Geometry: see drawing. Coordinates: mm, zero at the bounding-box minimum. Coordinates: 2 decimals unless noted, no trailing zeros. Order: outer loops, then holes, each group sorted by start corner. A loop starts at its lowest first (then second) coordinate and runs counter-clockwise, first axis right, second up.
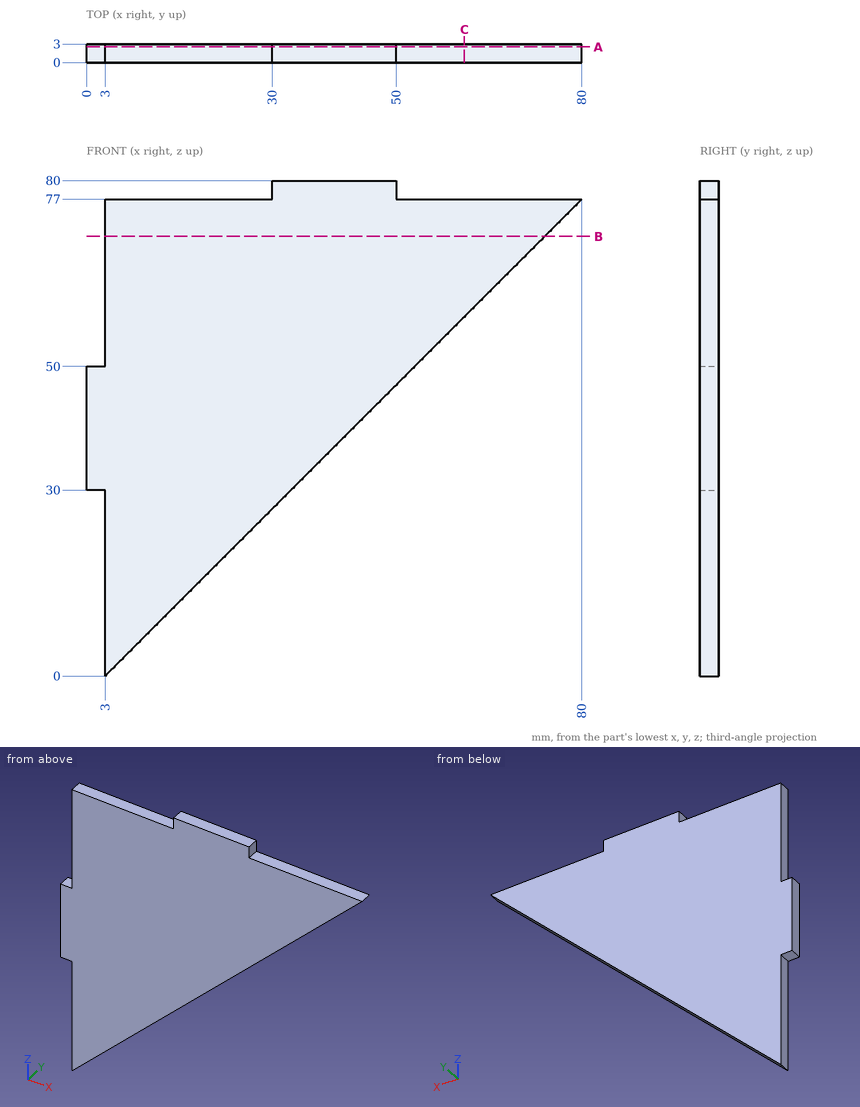
Q1. Section query C-C on x = 61. Output: boundary loops of the cut face in (y, z).
Solutions:
outline: (0, 58) - (3, 58) - (3, 77) - (0, 77) - close
Q2. Section query B-B on z = 71. Output: boundary loops of the cut face in (x, y).
Solutions:
outline: (3, 0) - (74, 0) - (74, 3) - (3, 3) - close
Q3. Pin query (flat end, axial travel): P1, Ø0.9, axis at y = 1, z = 78.5, coming from the +X side; P2, Ø1, axis at y = 0.5, z = 52.5, coming from the +X side; P3, Ø0.9, axis at x = 68.5, y = 1, coming from the +Z side. Return the tip coordinate at first contact, or that it passes through.
Solutions:
P1: stops at x = 50
P2: stops at x = 56
P3: stops at z = 77
Q4. Material intervals for line 1 along X through (y, z) = (2.5, 77.5); line 2 along Z through (x, y) = (36.5, 0.3); line 3 along X through (y, z) = (2.1, 38.5), sorted ascending.
Solutions:
line 1: x = 30 to 50
line 2: z = 33.5 to 80
line 3: x = 0 to 41.5
Q5. Section query A-A on y = 2.55. Output: boundary loops of the cut face in (x, z), plus the area to 3 significant figures.
Solutions:
outline: (0, 30) - (3, 30) - (3, 0) - (80, 77) - (50, 77) - (50, 80) - (30, 80) - (30, 77) - (3, 77) - (3, 50) - (0, 50) - close
area: 3,080 mm2
